```python
from build123d import *

# Parameters (mm, degrees)
SKETCH1_W           = 57.15
SKETCH1_H           = 31.75
BOSS_EXTRUDE1_DEPTH = 19.05
SKETCH2_W           = 57.15
SKETCH2_H           = 9.525
CUT_EXTRUDE1_DEPTH  = 0.635
SKETCH3_R           = 1.778
SKETCH3_R_2         = 1.8288
SKETCH3_R_3         = 2.1844
SKETCH3_R_4         = 2.4892
SKETCH3_R_5         = 3.2639
CUT_EXTRUDE2_DEPTH  = 38.518774967


with BuildPart() as part:
    # Sketch1 → Boss-Extrude1 (new body)
    with BuildSketch(Plane(origin=(0, 0, 0), x_dir=(1, 0, 0), z_dir=(0, 1, 0))):
        Rectangle(SKETCH1_W, SKETCH1_H)
    extrude(amount=BOSS_EXTRUDE1_DEPTH)

    # Sketch2 → Cut-Extrude1 (cut)
    with BuildSketch(Plane(origin=(0, 19.05, 0), x_dir=(1, 0, 0), z_dir=(0, 1, 0))):
        Rectangle(SKETCH2_W, SKETCH2_H)
    extrude(amount=-CUT_EXTRUDE1_DEPTH, mode=Mode.SUBTRACT)

    # Sketch3 → Cut-Extrude2 (cut, through all)
    with BuildSketch(Plane(origin=(0, 18.415, 0), x_dir=(1, 0, 0), z_dir=(0, 1, 0))):
        with Locations(Location((-19.05, 0, 0), (0, 0, 270))):
            Circle(SKETCH3_R)
        with Locations(Location((-9.525, 0, 0), (0, 0, 270))):
            Circle(SKETCH3_R_2)
        with Locations(Location((0, 0, 0), (0, 0, 270))):
            Circle(SKETCH3_R_3)
        with Locations(Location((9.525, 0, 0), (0, 0, 270))):
            Circle(SKETCH3_R_4)
        with Locations(Location((19.05, 0, 0), (0, 0, 270))):
            Circle(SKETCH3_R_5)
    extrude(amount=-CUT_EXTRUDE2_DEPTH, mode=Mode.SUBTRACT)


solid = part.part
```
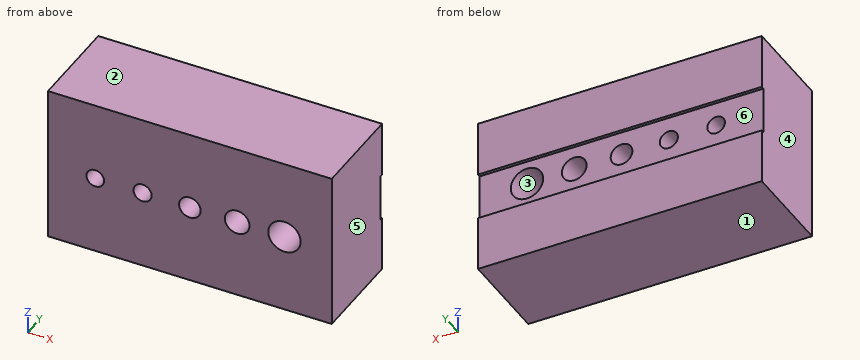
Design review of the part built by this model. Coordinates are the model's own, in mm. Face numbers are marked on the shaded views. A direction names the side the tool comes from. Coordinates: 2 decimals unless noted, no trailing zeros. Order: outer loops, then holes, each group sorted by start corner. A loop starts at its lowest first (then second) coordinate and runs counter-clockwise, first axis right, second up.
1) For the marked faces 5 and 6, list the 3-axis set-ups (+Z, -Z, +X, -X, +Y, -Y) from which the entire face can be reached by the end or side of a thin tool; tool diameter is ignored.
2) Take a section at A-A, the plane z = 0. Give the boundary of the cut face in (x, y) (3 decimals).
3) Mouldability with a two-part tool opening along Z and no side actions: class the marked faces 1, 2, 3 and 4 as +Z half, -Z half, draft (parallel to the pull), parting line (faces both ways), or undercut.
4) Take a section at C-C, the plane y = 9.5. Give the boundary of the cut face in (x, z) (3 decimals), and give its area (3 significant figures).
5) Wall thickness on line 1 along X through (y, z) = (4.5, 0) (3 decimals); line 2 along X through (y, z) = (8.5, -1) (1 decimal); line 3 along X through (y, z) = (3.5, -2) (3 decimals): over which ranges is each line inside the solid? List them lowest first.
6) Clearance check with a flat-ended pin moving along its axis: pin 1 (5 mm diameter, centred on x = 3.5, z = 0.5, fed in from +Y) (3 decimals). State where the tip first meets the part, or that it passes through.
Returned:
1. face 5: +Z, -Z, +X, +Y, -Y
1. face 6: +X, -X, +Y
2. outline: (-28.575, 0) - (-20.828, 0) - (-20.828, 18.415) - (-28.575, 18.415) - close; (-17.272, 0) - (-11.354, 0) - (-11.354, 18.415) - (-17.272, 18.415) - close; (-7.696, 0) - (-2.184, 0) - (-2.184, 18.415) - (-7.696, 18.415) - close; (2.184, 0) - (7.036, 0) - (7.036, 18.415) - (2.184, 18.415) - close; (12.014, 0) - (15.786, 0) - (15.786, 18.415) - (12.014, 18.415) - close; (22.314, 0) - (28.575, 0) - (28.575, 18.415) - (22.314, 18.415) - close
3. face 1: -Z half
3. face 2: +Z half
3. face 3: undercut
3. face 4: draft
4. outline: (-28.575, -15.875) - (28.575, -15.875) - (28.575, 15.875) - (-28.575, 15.875) - close; hole circle Ø3.556 at (-19.05, 0); hole circle Ø3.658 at (-9.525, 0); hole circle Ø4.369 at (0, 0); hole circle Ø4.978 at (9.525, 0); hole circle Ø6.528 at (19.05, 0)
4. area: 1,730 mm2
5. line 1: x = -28.575 to -20.828, -17.272 to -11.354, -7.696 to -2.184, 2.184 to 7.036, 12.014 to 15.786, 22.314 to 28.575
5. line 2: x = -28.6 to -20.5, -17.6 to -11.1, -8 to -1.9, 1.9 to 7.2, 11.8 to 15.9, 22.2 to 28.6
5. line 3: x = -28.575 to -0.878, 0.878 to 8.043, 11.007 to 16.471, 21.629 to 28.575
6. pin 1: stops at y = 18.415
